Study the drawing (mm; zero at the part's minimum x, y, z) and answer. Coordinates: 2 decimals unless noted, no trailing zeros. Order: outer loops, then holes, each group sorted by start corner. A loop starts at its lowest first (then second) coordinate and runs counter-clockwise, first axis right, second up.
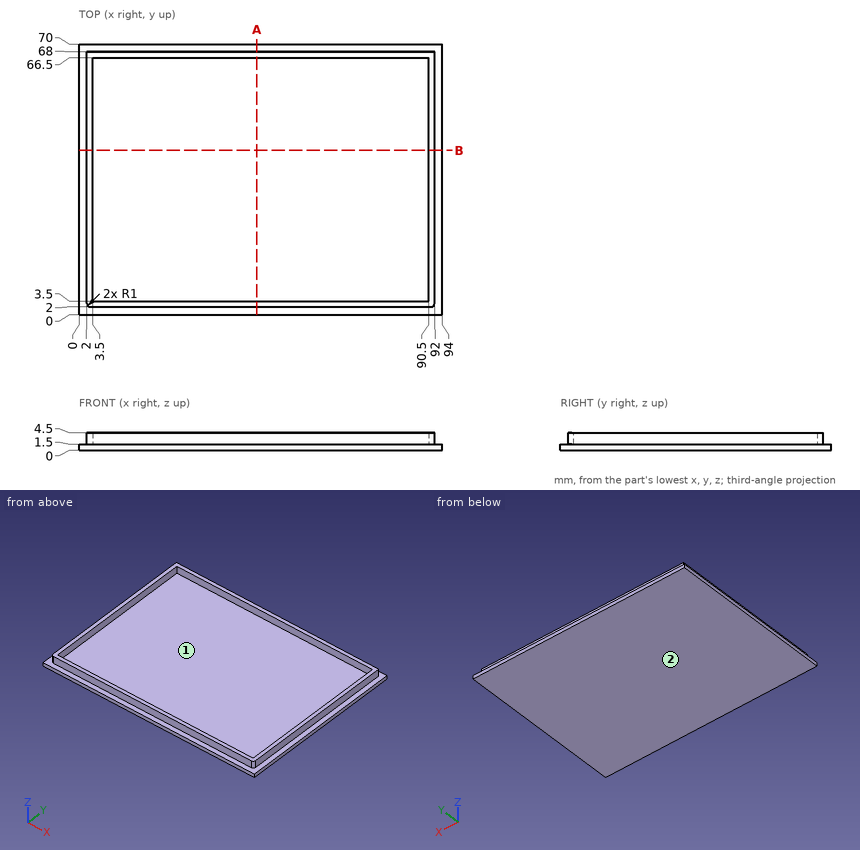
(1) Find section A-A (x = 46). Write down the section's boundary in (y, z).
(2) Each of these flat-tipped pins is pushed along its axis until it touches: pin 1 Ø1.5 at (x, z) = (29, 2.5) entering from -Y; pin 2 Ø1.5 at (y, z) = (26.5, 3.5) entering from -X; pin 3 Ø2.5 at (y, z) = (32.5, 3.5) entering from +X; pin 4 Ø2.5 at (y, z) = (22.5, 2.5) entering from -X. Where does it stop, or does it pass through?
(3) Find section B-B (y = 42.5). Write down the section's boundary in (x, z).
(4) The mould has two halves that part along Y. Classify the marked faces 1 and 2: released by +Y, released by -Y, zero draft, split by the parting line, or undercut.
(5) Consider line 1 (Y direction, x = 42, z = 1.6); line 2 (X direction, y = 61, z = 3.85); line 3 (Z direction, x = 55.5, y = 50.5). Determine where each line is inside the solid, lowest interval first.
Findings below:
1. outline: (0, 0) - (70, 0) - (70, 1.5) - (68, 1.5) - (68, 4.5) - (66.5, 4.5) - (66.5, 1.5) - (3.5, 1.5) - (3.5, 4.5) - (2, 4.5) - (2, 1.5) - (0, 1.5) - close
2. pin 1: stops at y = 2
2. pin 2: stops at x = 2
2. pin 3: stops at x = 92
2. pin 4: stops at x = 0
3. outline: (0, 0) - (94, 0) - (94, 1.5) - (92, 1.5) - (92, 4.5) - (90.5, 4.5) - (90.5, 1.5) - (3.5, 1.5) - (3.5, 4.5) - (2, 4.5) - (2, 1.5) - (0, 1.5) - close
4. face 1: undercut
4. face 2: zero draft
5. line 1: y = 2 to 3.5, 66.5 to 68
5. line 2: x = 2 to 3.5, 90.5 to 92
5. line 3: z = 0 to 1.5
